Can you work these out from the model? Positions are in its coordinate system, mm. A direction names the side the tool comes from. Give positions to 0.01 mm unless a question says otherwise; leave off trailing zeros. Order: outer loops, then holes, each group sorted by start corner. A loop starts at its lowest first (then second) coordinate and runs counter-clockwise, first axis right, second up. Notation, with made-up numbers: (-36, -19.5) - (-25, -19.5) arc R15 cw to (-25, -15.5) - close; hole circle Ø3 at (57, -29). An arc over 180 degrees is marked (long way). Answer as CSV lines item,"result".
```python
from build123d import *

# Parameters (mm, degrees)
SKETCH1_R                = 15
BOSS_EXTRUDE1_DEPTH      = 20
SKETCH2_R                = 10.95
BOSS_EXTRUDE2_DEPTH      = 3.5
SKETCH4_R                = 3.05
CUT_EXTRUDE1_DEPTH       = 4.1
SKETCH5_R                = 1.5
CUT_EXTRUDE2_DEPTH       = 4
SKETCH7_R                = 10.95
SKETCH7_R_2              = 3
BOSS_EXTRUDE3_DEPTH      = 11
SKETCH9_R                = 1.5
CUT_EXTRUDE4_DEPTH       = 41.5
BOSS_EXTRUDE4_START      = 7
SKETCH12_R               = 18
SKETCH12_R_2             = 3.25
SKETCH12_R_3             = 3.05
BOSS_EXTRUDE4_DEPTH      = 7
CUT_EXTRUDE9_START       = -5
SKETCH13_R               = 1.5
CUT_EXTRUDE9_DEPTH       = 17
CIRPATTERN1_COUNT        = 3
CUT_EXTRUDE12_DEPTH      = 15
CUT_EXTRUDE12_DEPTH_BACK = 38.1079508
SKETCH15_R               = 13
SKETCH15_R_2             = 10.95
BOSS_EXTRUDE6_START      = 13
SKETCH17_R               = 13
BOSS_EXTRUDE6_DEPTH      = 20
SKETCH19_R               = 2.5
CUT_EXTRUDE13_DEPTH      = 38.107950728
SKETCH20_R               = 5
SKETCH20_R_2             = 2.5
CUT_EXTRUDE14_DEPTH      = 5


with BuildPart() as part:
    # Sketch1 → Boss-Extrude1 (new body)
    with BuildSketch(Plane.XY):
        Circle(SKETCH1_R)
    extrude(amount=BOSS_EXTRUDE1_DEPTH)

    # Sketch2 → Boss-Extrude2 (add)
    with BuildSketch(Plane.XY.offset(20)):
        Circle(SKETCH2_R)
    extrude(amount=BOSS_EXTRUDE2_DEPTH)

    # Sketch4 → Cut-Extrude1 (cut)
    with BuildSketch(Plane(origin=(0, 0, 0), x_dir=(-1, 0, 0), z_dir=(0, 0, -1))):
        Circle(SKETCH4_R)
    extrude(amount=-CUT_EXTRUDE1_DEPTH, mode=Mode.SUBTRACT)

    # Sketch5 → Cut-Extrude2 (cut)
    with BuildSketch(Plane(origin=(0, 0, 4.1), x_dir=(-1, 0, 0), z_dir=(0, 0, -1))):
        Circle(SKETCH5_R)
    extrude(amount=-CUT_EXTRUDE2_DEPTH, mode=Mode.SUBTRACT)

    # Sketch7 → Boss-Extrude3 (add)
    with BuildSketch(Plane.XY.offset(23.5)):
        Circle(SKETCH7_R)
        Circle(SKETCH7_R_2, mode=Mode.SUBTRACT)
    extrude(amount=BOSS_EXTRUDE3_DEPTH)

    # Sketch9 → Cut-Extrude4 (cut, through all)
    with BuildSketch(Plane.XY.offset(34.5)):
        with Locations((7, 0)):
            Circle(SKETCH9_R)
        with Locations((-3.5, -6.062177826)):
            Circle(SKETCH9_R)
        with Locations((-3.5, 6.062177826)):
            Circle(SKETCH9_R)
    extrude(amount=-CUT_EXTRUDE4_DEPTH, mode=Mode.SUBTRACT)

    # Sketch12 → Boss-Extrude4 (add)
    with BuildSketch(Plane(origin=(0, 0, 0), x_dir=(-1, 0, 0), z_dir=(0, 0, -1)).offset(BOSS_EXTRUDE4_START)):
        Circle(SKETCH12_R)
        with Locations((3.5, 6.062177826)):
            Circle(SKETCH12_R_2, mode=Mode.SUBTRACT)
        with Locations((3.5, -6.062177826)):
            Circle(SKETCH12_R_2, mode=Mode.SUBTRACT)
        with Locations((-7, 0)):
            Circle(SKETCH12_R_2, mode=Mode.SUBTRACT)
        Circle(SKETCH12_R_3, mode=Mode.SUBTRACT)
    extrude(amount=-BOSS_EXTRUDE4_DEPTH)

    # Sketch13 → Cut-Extrude9 (cut)
    with BuildSketch(Plane(origin=(0, 0, 0), x_dir=(0, 0, -1), z_dir=(1, 0, 0)).offset(CUT_EXTRUDE9_START)):
        with Locations((2, 0)):
            Circle(SKETCH13_R)
    cut_extrude9 = extrude(amount=-CUT_EXTRUDE9_DEPTH, mode=Mode.SUBTRACT)

    # CirPattern1: Cut-Extrude9 ×3 about axis
    cirpattern1_axis = Axis((0, 0, 0), (0, 0, 1))
    for i in range(1, CIRPATTERN1_COUNT):
        add(cut_extrude9.rotate(cirpattern1_axis, i * 360 / CIRPATTERN1_COUNT), mode=Mode.SUBTRACT)

    # Sketch15 → Cut-Extrude12 (cut, two sides: drawn at the far end of the back side and taken through both)
    # profile 1 of 2: a face of its own
    with BuildSketch(Plane.XY.offset(20).offset(-CUT_EXTRUDE12_DEPTH_BACK)):
        Circle(SKETCH15_R)
        Circle(SKETCH15_R_2, mode=Mode.SUBTRACT)
    # profile 2 of 2: a face of its own
    with BuildSketch(Plane.XY.offset(20).offset(-CUT_EXTRUDE12_DEPTH_BACK)):
        Circle(SKETCH15_R_2)
    extrude(amount=CUT_EXTRUDE12_DEPTH + CUT_EXTRUDE12_DEPTH_BACK, mode=Mode.SUBTRACT)

    # Sketch17 → Boss-Extrude6 (add)
    with BuildSketch(Plane.XY.offset(BOSS_EXTRUDE6_START)):
        Circle(SKETCH17_R)
    extrude(amount=-BOSS_EXTRUDE6_DEPTH)

    # Sketch19 → Cut-Extrude13 (cut, through all)
    with BuildSketch(Plane(origin=(0, 0, -7), x_dir=(-1, 0, 0), z_dir=(0, 0, -1))):
        with Locations((7.66, 0)):
            Circle(SKETCH19_R)
        with Locations((-3.83, -6.633754593)):
            Circle(SKETCH19_R)
        with Locations((-3.83, 6.633754593)):
            Circle(SKETCH19_R)
    extrude(amount=-CUT_EXTRUDE13_DEPTH, mode=Mode.SUBTRACT)

    # Sketch20 → Cut-Extrude14 (cut)
    # profile 1 of 3: a face of its own
    with BuildSketch(Plane(origin=(0, 0, -7), x_dir=(-1, 0, 0), z_dir=(0, 0, -1))):
        with Locations((7.66, 0)):
            Circle(SKETCH20_R)
        with Locations((7.66, 0)):
            Circle(SKETCH20_R_2, mode=Mode.SUBTRACT)
    # profile 2 of 3: a face of its own
    with BuildSketch(Plane(origin=(0, 0, -7), x_dir=(-1, 0, 0), z_dir=(0, 0, -1))):
        with Locations((-3.83, 6.633754593)):
            Circle(SKETCH20_R)
        with Locations((-3.83, 6.633754593)):
            Circle(SKETCH20_R_2, mode=Mode.SUBTRACT)
    # profile 3 of 3: a face of its own
    with BuildSketch(Plane(origin=(0, 0, -7), x_dir=(-1, 0, 0), z_dir=(0, 0, -1))):
        with Locations((-3.83, -6.633754593)):
            Circle(SKETCH20_R)
        with Locations((-3.83, -6.633754593)):
            Circle(SKETCH20_R_2, mode=Mode.SUBTRACT)
    extrude(amount=-CUT_EXTRUDE14_DEPTH, mode=Mode.SUBTRACT)


solid = part.part
```
1) I want a section at A-A on y = 0. Write out the boundary of the cut face in (x, z).
Answer block:
outline,"(-18, -7) - (-12.66, -7) - (-12.66, -2) - (-10.16, -2) - (-10.16, 13) - (-13, 13) - (-13, 20) - (-15, 20) - (-15, 0) - (-18, 0) - (-18, -0.5) - (-13, -0.5) - (-13, -3.5) - (-18, -3.5) - close; (-5.16, -2) - (-2.66, -2) - (-2.66, -7) - (18, -7) - (18, 0) - (15, 0) - (15, 20) - (13, 20) - (13, 13) - (-5.16, 13) - close"
2) I need wall thicknesses on line 1 along Y through (x, z) = (3.83, 3.5); line 2 along Y through (x, z) = (0, 14.75); line 3 along Y through (x, z) = (3.83, -4.3). Which ranges of each line are inside material? Lowest first, please. Write a range as [from, to].
Answer block:
line 1,"[-14.5, -9.13], [-4.13, 4.13], [9.13, 14.5]"
line 2,"[-15, -13], [13, 15]"
line 3,"[-17.59, -11.63], [-1.63, 1.63], [11.63, 17.59]"
3) If we mould it in two halves opening along Z, with no side actions, what happens to faces 1 (the cylindrical face through (-10.316, -7.91, 16.451)), 2 (the cylindrical face through (-15.42, 0.07, -0.5)), 3 (the flat face through (-5, -1, -2))? For each: +Z half, -Z half, draft (parallel to the pull), parting line (faces both ways), or undercut.
Answer block:
face 1,"draft"
face 2,"undercut"
face 3,"-Z half"
4) I'm going to push flat-ended pins straight in: P1, Ø8, axis at x = 3.83, y = -6.63, coming from the +Z side; P2, Ø10, axis at x = 13.5, z = 11, coming from the +Y side; P3, Ø3, axis at x = 6, y = -8, coming from the -Z side. Where does each tip first touch, or does it pass through?
Answer block:
P1,"z = 13"
P2,"y = 12.36"
P3,"z = -2"
5) I want a section at C-C on z = -2.75. Write out the boundary of the cut face in (x, y), plus the area to 3 significant figures.
Answer block:
outline,"(-17.95, -1.3) arc R18 ccw to (7.85, -16.2) - (5.34, -11.85) arc R13 ccw to (7.59, -10.55) - (10.1, -14.9) arc R18 ccw to (10.1, 14.9) - (7.59, 10.55) arc R13 ccw to (5.34, 11.85) - (7.85, 16.2) arc R18 ccw to (-17.95, 1.3) - (-12.93, 1.3) arc R13 ccw to (-12.93, -1.3) - close; hole circle Ø10 at (-7.66, 0); hole circle Ø10 at (3.83, -6.63); hole circle Ø10 at (3.83, 6.63)"
area,"743 mm2"
6) I want a section at D-D on x = 12.5. Write out the boundary of the cut face in (y, z).
Answer block:
outline,"(-12.95, -7) - (12.95, -7) - (12.95, 0) - (8.29, 0) - (8.29, 20) - (3.57, 20) - (3.57, 13) - (-3.57, 13) - (-3.57, 20) - (-8.29, 20) - (-8.29, 0) - (-12.95, 0) - close"
7) I want a section at B-B on x = 3.83. Write out the boundary of the cut face in (y, z), plus the area to 3 significant figures.
Answer block:
outline,"(-17.59, -7) - (-11.63, -7) - (-11.63, -2) - (-9.13, -2) - (-9.13, 13) - (-12.42, 13) - (-12.42, 20) - (-14.5, 20) - (-14.5, 0) - (-17.59, 0) - close; (-4.13, -2) - (-1.63, -2) - (-1.63, -7) - (1.63, -7) - (1.63, -2) - (4.13, -2) - (4.13, 13) - (-4.13, 13) - close; (9.13, -2) - (11.63, -2) - (11.63, -7) - (17.59, -7) - (17.59, 0) - (14.5, 0) - (14.5, 20) - (12.42, 20) - (12.42, 13) - (9.13, 13) - close"
area,"402 mm2"
8) Which directions (+Z, -Z, +X, -X, +Y, -Y) give clear straight access to the entire face, cutting with the end or side of a thin tool? Please do faces 4 (the cylindrical face through (6.48, -11.27, -1.97)), 5 (the flat face through (2, 4, -2)), 6 (the cylindrical face through (-14.985, 0.66, 9.86)).
Answer block:
face 4,"none"
face 5,"-Z"
face 6,"+Z"
